```python
from build123d import *

# Parameters (mm, degrees)
BOSS_EXTRUDE1_DEPTH      = 75
BOSS_EXTRUDE1_DEPTH_BACK = 75
SKETCH4_R                = 50
CUT_EXTRUDE1_DEPTH       = 50


with BuildPart() as part:
    # Sketch2 → Boss-Extrude1 (new, two sides: drawn at the far end of the back side and taken through both)
    with BuildSketch(Plane(origin=(0, 0, 0), x_dir=(0, 0, -1), z_dir=(1, 0, 0)).offset(-BOSS_EXTRUDE1_DEPTH_BACK)):
        Polygon((75, 25), (50, 25), (50, 50), (25, 50), (25, 25), (0, 25), (0, -25), (25, -25), (25, -50), (50, -50), (50, -25), (75, -25), (75, -75), (-75, -75), (-75, 75), (75, 75), align=None)
    extrude(amount=BOSS_EXTRUDE1_DEPTH + BOSS_EXTRUDE1_DEPTH_BACK)

    # Sketch4 → Cut-Extrude1 (cut)
    with BuildSketch(Plane.XY.offset(75)):
        Circle(SKETCH4_R)
    extrude(amount=-CUT_EXTRUDE1_DEPTH, mode=Mode.SUBTRACT)


solid = part.part
```
The listing builds one solid part. Answer for the finished solid, in the listing's coordinates (mm). A direction names the side the tool comes from. Give positions to 0.01 mm unless a question says otherwise; leave off trailing zeros. Order: outer loops, then holes, each group sorted by start corner. A loop starts at its lowest first (then second) coordinate and runs counter-clockwise, first axis right, second up. Notation, with made-up numbers: (-7, -3) - (9, -3) arc R10 cw to (9, 10) - close; hole circle Ø8 at (74, 20.25). An arc over 180 degrees is marked (long way). Answer in a Markdown table with one row per item. Add a question column.
Q1. The part is cut by section C-C (y = 46). Determine the outline of the cut face in (x, z).
Q2. For a pull along Y with two mould halves and no side action, classify faces 5 (the flat face through (-1, -75, -1)), 6 (the flat face through (-1, -50, -75)), 7 (the flat face through (-1, 1, 25)), 8 (the flat face through (-1, 50, -38)) as released by +Y, released by -Y, zero draft, split by the parting line, or undercut.
Q3. The part is cut by section B-B (x = 54.5). Determine the outline of the cut face in (y, z), then the cut area to 3 significant figures.
Q4. The part is cut by section D-D (z = 56). Determine the outline of the cut face in (x, y).
Q5. The part is cut by section A-A (z = -38.5). Determine the outline of the cut face in (x, y), then the cut area to 3 significant figures.
Q6. Find the intervals of material crossed by line 1 along Y through (x, z) = (0, 45.5); line 2 along Y through (x, z) = (17, -62.5); line 3 along Z through (x, y) = (43.5, 6.5), in increasing order. Write a range as [from, to].
Q7. Which of the six approach directions +Z, -Z, +X, -X, +Y, -Y give full straight-line access (tool end or side, diameter ignored) to faces 1 (the flat face through (-1, 75, 1)), 2 (the flat face through (-1, 38, -25)), 3 (the cylindrical face through (47.69, 15.02, 50.35)), 4 (the flat face through (-1, 0, 0))?
Q8. Given P1, Ø5, axis at x = 11, y = 11, coming from the +Z side, flat-ended and moving along its own axis, determine where the tip first touches the part or whether it passes through.
Determined:
| question | item | result |
|---|---|---|
| 1 | outline | (-75, -75) - (75, -75) - (75, -50) - (-75, -50) - close; (-75, -25) - (75, -25) - (75, 75) - (19.6, 75) - (19.6, 25) - (-19.6, 25) - (-19.6, 75) - (-75, 75) - close |
| 2 | face 5 | released by -Y |
| 2 | face 6 | zero draft |
| 2 | face 7 | undercut |
| 2 | face 8 | undercut |
| 3 | outline | (-75, -75) - (-25, -75) - (-25, -50) - (-50, -50) - (-50, -25) - (-25, -25) - (-25, 0) - (25, 0) - (25, -25) - (50, -25) - (50, -50) - (25, -50) - (25, -75) - (75, -75) - (75, 75) - (-75, 75) - close |
| 3 | area | 17,500 mm² |
| 4 | outline | (-75, -75) - (75, -75) - (75, 75) - (-75, 75) - close; hole circle Ø100 at (0, 0) |
| 5 | outline | (-75, -75) - (75, -75) - (75, -50) - (-75, -50) - close; (-75, 50) - (75, 50) - (75, 75) - (-75, 75) - close |
| 5 | area | 7,500 mm² |
| 6 | line 1 | y = [-75, -50], [50, 75] |
| 6 | line 2 | y = [-75, -25], [25, 75] |
| 6 | line 3 | z = [0, 25] |
| 7 | face 1 | +Z, -Z, +X, -X, +Y |
| 7 | face 2 | +X, -X |
| 7 | face 3 | +Z |
| 7 | face 4 | -Z, +X, -X |
| 8 | P1 | stops at z = 25 |
